Input: part model. Units: mm. Frame: model coordinates. A direction names the side the tool comes from. Give positions to 0.01 mm unless a question says otherwise; leave off trailing zeros. Write each loop counter-clockwise with the first axis right and the second up, starting at its lowest first coordinate (ties: lowest second). Pieces come first, ordered by that corner, then holes. Notation, with made-up numbers: (85.25, -14.5) -> (93.25, -14.5) arc R11 ccw to (93.25, -3.5) -> close; hole circle Ø11 at (-1.75, -13). An arc over 180 degrees is marked (long way). Return JSON: item names as keys, results as strings. Group by question number.
Item 1: Section B-B, the plane z = -2.5. Return loops of the section in (x, y).
Item 2: Set-up query: faces 1 (the face through (12.138, 8.618, -1.521)), 2 (the face through (1.382, -0.496, -3.362)), 3 (the face through (-7.313, -10.638, -3.382)), 4 (the face through (0, -12, -12)), 5 (the face through (-9.55, -11.49, -5.46)). Return all of +Z, -Z, +X, -X, +Y, -Y with unobstructed straight access to the full face (end or side cutting, diameter ignored); none if empty.
Item 3: Pin query (flat end, axial travel): P1, Ø4.5, axis at x = -7, z = -8, coming from the +Y side; P2, Ø5, axis at x = 8.5, z = -8, coming from the +Y side; P3, Ø3.5, axis at y = -4, z = -9, coming from the +X side. Return the tip coordinate at first contact, or that it passes through.
Item 4: Mould query, pull axis X, two halves, no side actions, for faces 6 (the face through (-11, -6, -1)), 7 (the face through (7, 0, -3)), 8 (the face through (-1, -5, -6)), 9 (the face through (1.382, -10.638, -8.189)). Classes: released by +X, released by -X, zero draft, split by the parting line, or undercut.
Item 5: Line query: line 1 (X direction, y = -12.7, z = -8); line 2 (Y direction, x = -10.5, z = -1.3); line 3 (X direction, y = -11.75, z = -8). Output: solid intervals per line, ascending. Write a range as [from, to].
Item 6: Section C-C, the plane y = -6.75. Return loops of the section in (x, z).
Item 7: Section D-D, the plane x = 5. Return loops of the section in (y, z), then the cut area to 3 significant figures.
Item 8: Section A-A, the plane x = -8.5. Return loops of the section in (y, z), then the cut area to 3 significant figures.
from build123d import *

# Parameters (mm, degrees)
SKETCH1_W                       = 25
SKETCH1_H                       = 23
SKETCH1_R                       = 0.9
BOSS_EXTRUDE1_DEPTH             = 3
BOSS_EXTRUDE2_REACH             = 21.007
BOSS_EXTRUDE2_DIRECTION_2_REACH = 21.007
SKETCH3_W                       = 11.5
SKETCH3_H                       = 9
CUT_EXTRUDE1_DEPTH              = 20
SKETCH4_R                       = 1.6
CUT_EXTRUDE2_DEPTH              = 27.462237245
SKETCH5_R                       = 2.75
CUT_EXTRUDE3_DEPTH              = 1
FILLET2_R                       = 1.27


with BuildPart() as part:
    # Sketch1 → Boss-Extrude1 (new body)
    with BuildSketch(Plane.XY):
        with Locations((0, -2.5)):
            Rectangle(SKETCH1_W, SKETCH1_H)
        with Locations((-10.5, 6.75)):
            Circle(SKETCH1_R, mode=Mode.SUBTRACT)
        with Locations((10.5, 6.75)):
            Circle(SKETCH1_R, mode=Mode.SUBTRACT)
        with Locations((10.5, -6.75)):
            Circle(SKETCH1_R, mode=Mode.SUBTRACT)
        with Locations((-10.5, -6.75)):
            Circle(SKETCH1_R, mode=Mode.SUBTRACT)
    extrude(amount=-BOSS_EXTRUDE1_DEPTH)

    # Boss-Extrude2: up to this face of the body (flat: up to its plane)
    boss_extrude2_end = Plane(part.part.faces().sort_by_distance((12.5, -2.5, -1.5))[0])
    # Sketch2 → Boss-Extrude2 (add, up to the picked face)
    with BuildSketch(Plane(origin=(0, 0, 0), x_dir=(0, 0, -1), z_dir=(1, 0, 0)), mode=Mode.PRIVATE) as boss_extrude2_sk1:
        Polygon((3, 9), (12, -11), (12, -14), (3, -14), align=None)
    boss_extrude2_tool1 = split(extrude(boss_extrude2_sk1.sketch, amount=BOSS_EXTRUDE2_REACH, mode=Mode.PRIVATE), bisect_by=boss_extrude2_end, keep=Keep.BOTH, mode=Mode.PRIVATE)
    add(boss_extrude2_tool1.solids().sort_by(Axis((0, -6.217949, -6.346154), (1, 0, 0)))[0])

    # Boss-Extrude2 direction 2: up to this face of the body (flat: up to its plane)
    boss_extrude2_direction_2_end = Plane(part.part.faces().sort_by_distance((-12.5, -2.5, -1.5))[0])
    # Sketch2 → Boss-Extrude2 direction 2 (add, up to the picked face)
    with BuildSketch(Plane(origin=(0, 0, 0), x_dir=(0, 0, -1), z_dir=(1, 0, 0)), mode=Mode.PRIVATE) as boss_extrude2_direction_2_sk1:
        Polygon((3, 9), (12, -11), (12, -14), (3, -14), align=None)
    boss_extrude2_direction_2_tool1 = split(extrude(boss_extrude2_direction_2_sk1.sketch, amount=-BOSS_EXTRUDE2_DIRECTION_2_REACH, mode=Mode.PRIVATE), bisect_by=boss_extrude2_direction_2_end, keep=Keep.BOTH, mode=Mode.PRIVATE)
    add(boss_extrude2_direction_2_tool1.solids().sort_by(Axis((0, -6.217949, -6.346154), (-1, 0, 0)))[0])

    # Sketch3 → Cut-Extrude1 (cut)
    with BuildSketch(Plane(origin=(0, 9, 0), x_dir=(1, 0, 0), z_dir=(0, 1, 0))):
        with Locations((-6.75, 7.5)):
            Rectangle(SKETCH3_W, SKETCH3_H)
        with Locations((6.75, 7.5)):
            Rectangle(SKETCH3_W, SKETCH3_H)
    extrude(amount=-CUT_EXTRUDE1_DEPTH, mode=Mode.SUBTRACT)

    # Sketch4 → Cut-Extrude2 (cut, through all)
    with BuildSketch(Plane(origin=(0, -11, 0), x_dir=(1, 0, 0), z_dir=(0, 1, 0))):
        with Locations(Location((-8.5, 8, 0), (0, 0, 270))):
            Circle(SKETCH4_R)
        with Locations(Location((8.5, 8, 0), (0, 0, 90))):
            Circle(SKETCH4_R)
    extrude(amount=-CUT_EXTRUDE2_DEPTH, mode=Mode.SUBTRACT)

    # Sketch5 → Cut-Extrude3 (cut)
    with BuildSketch(Plane(origin=(0, -11, 0), x_dir=(1, 0, 0), z_dir=(0, 1, 0))):
        with Locations(Location((-8.5, 8, 0), (0, 0, 270))):
            Circle(SKETCH5_R)
        with Locations(Location((8.5, 8, 0), (0, 0, 270))):
            Circle(SKETCH5_R)
    extrude(amount=-CUT_EXTRUDE3_DEPTH, mode=Mode.SUBTRACT)

    # Fillet2
    fillet2_edges = [part.edges().sort_by_distance(p)[0] for p in [
        (-12.5, -12.5, -12),
        (12.5, -12.5, -12),
        (-1, -11, -7.5),
        (-6.75, -11, -3),
        (-1, -1, -3),
        (1, -1, -3),
        (1, -11, -7.5),
        (6.75, -11, -3),
        (-12.5, 9, -1.5),
        (12.5, 9, -1.5),
    ]]
    fillet(fillet2_edges, radius=FILLET2_R)


solid = part.part
Answer below:
{
 "1": {"outline": "(-12.5, -14) -> (12.5, -14) -> (12.5, 7.73) arc R1.27 ccw to (11.23, 9) -> (-11.23, 9) arc R1.27 ccw to (-12.5, 7.73) -> close; hole circle Ø1.8 at (-10.5, -6.75); hole circle Ø1.8 at (-10.5, 6.75); hole circle Ø1.8 at (10.5, -6.75); hole circle Ø1.8 at (10.5, 6.75)"},
 "2": {"face 1": "+Z, -Z, +X, +Y", "face 2": "-Z, +X, +Y", "face 3": "-Z, -X, +Y", "face 4": "-Z, +X, -X, +Y, -Y", "face 5": "+Y"},
 "3": {"P1": "stops at y = -11", "P2": "stops at y = -12", "P3": "stops at x = 1"},
 "4": {"face 6": "undercut", "face 7": "zero draft", "face 8": "released by -X", "face 9": "released by +X"},
 "5": {"line 1": "x = [-12.5, -10.1], [-6.9, 6.9], [10.1, 12.5]", "line 2": "y = [-14, -7.65], [-5.85, 5.85], [7.65, 9]", "line 3": "x = [-12.5, -11.25], [-5.75, 5.75], [11.25, 12.5]"},
 "6": {"outline": "(-12.5, -3) -> (-11.4, -3) -> (-11.4, 0) -> (-12.5, 0) -> close; (-9.6, -3) -> (-2.27, -3) arc R1.27 cw to (-1, -4.27) -> (-1, -10.09) -> (1, -10.09) -> (1, -4.27) arc R1.27 cw to (2.27, -3) -> (9.6, -3) -> (9.6, 0) -> (-9.6, 0) -> close; (11.4, -3) -> (12.5, -3) -> (12.5, 0) -> (11.4, 0) -> close"},
 "7": {"outline": "(-14, -12) -> (-11, -12) -> (-11, -4.27) arc R1.27 cw to (-9.73, -3) -> (9, -3) -> (9, 0) -> (-14, 0) -> close", "area": "96.3 mm2"},
 "8": {"outline": "(-14, -12) -> (-11, -12) -> (-11, -10.75) -> (-12, -10.75) -> (-12, -9.6) -> (-14, -9.6) -> close; (-14, -6.4) -> (-12, -6.4) -> (-12, -5.25) -> (-11, -5.25) -> (-11, -4.27) arc R1.27 cw to (-9.73, -3) -> (9, -3) -> (9, 0) -> (-14, 0) -> close", "area": "84.4 mm2"}
}
